The listing builds one solid part. Answer for the finished solid, in the listing's coordinates (mm). Coordinates: 2 decimals unless noted, no trailing zeros. Loops run counter-clockwise (first coordinate to the right, second up) from the corner with the lowest first, then second, coordinate; pieces in that order, holes last. Notation, with made-up numbers: (15, 3.5) - (64, 3.5) arc R33 cw to (64, 33.5) - close; hole circle Ø4 at (67.5, 52.25). An arc over 180 degrees is marked (long way). One line per question, with ' | ' between items.
from build123d import *

# Parameters (mm, degrees)
SKETCH1_R           = 13.2
SKETCH1_R_2         = 6
BOSS_EXTRUDE1_DEPTH = 6
CUT_EXTRUDE1_DEPTH  = 7


with BuildPart() as part:
    # Sketch1 → Boss-Extrude1 (new body)
    with BuildSketch(Plane.XY):
        Circle(SKETCH1_R)
        Circle(SKETCH1_R_2, mode=Mode.SUBTRACT)
    extrude(amount=BOSS_EXTRUDE1_DEPTH)

    # Sketch2 → Cut-Extrude1 (cut, through all)
    with BuildSketch(Plane.XY.offset(6)):
        with BuildLine():
            ThreePointArc((-2.819851171, 12.895287487), (0, 13.2), (2.819851171, 12.895287487))
            ThreePointArc((2.819851171, 12.895287487), (1.826256171, 11.910750525), (1.819851171, 10.512))
            ThreePointArc((1.819851171, 10.512), (0, 10.668364555), (-1.819851171, 10.512))
            ThreePointArc((-1.819851171, 10.512), (-1.826256171, 11.910750525), (-2.819851171, 12.895287487))
        make_face()
    extrude(amount=-CUT_EXTRUDE1_DEPTH, mode=Mode.SUBTRACT)


solid = part.part
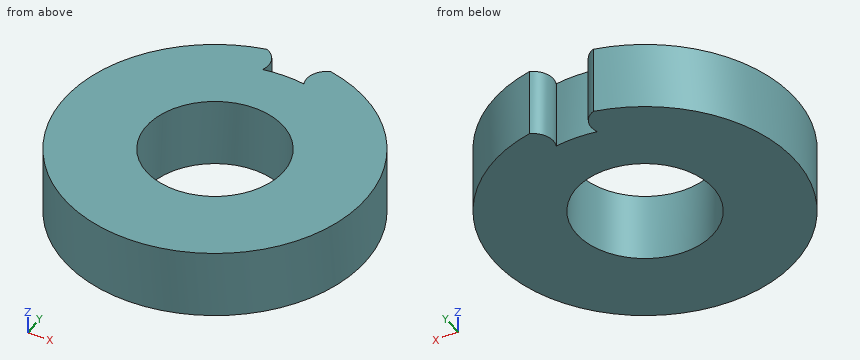
Item 1: Each of these flat-tipped pins is pushed along its axis until it touches: pin 1 Ø11 at (x, y) = (0, 0) entering from +Z; pin 2 Ø3 at (x, z) = (7, 0.5) entering from +Y; pin 3 Ø2 at (y, z) = (-4, 2) entering from -X; pin 4 Ø2 at (x, z) = (-1.5, 5) entering from +Y. Where does it stop, or does it pass through?
Taken from the geometry:
pin 1: passes through | pin 2: stops at y = 12 | pin 3: stops at x = -12.85 | pin 4: stops at y = 12.73
Item 2: Find section B-B, the plane y = 0. Write down the section's boundary in (x, z), plus the area to 3 significant figures.
Taken from the geometry:
outline: (-13.2, 0) - (-6, 0) - (-6, 6) - (-13.2, 6) - close; (6, 0) - (13.2, 0) - (13.2, 6) - (6, 6) - close | area: 86.4 mm2
Item 3: Find section D-D, the plane y = 6.75. Write down the section's boundary in (x, z), plus the area to 3 significant figures.
Taken from the geometry:
outline: (-11.34, 0) - (11.34, 0) - (11.34, 6) - (-11.34, 6) - close | area: 136 mm2
Item 4: Find section C-C, the plane z = 2.3. Write down the section's boundary in (x, y), plus the area to 3 significant figures.
Taken from the geometry:
outline: (-2.82, 12.9) arc R13.2 ccw (long way) to (2.82, 12.9) arc R1.83 ccw to (1.82, 10.51) arc R10.67 ccw to (-1.82, 10.51) arc R1.83 ccw to start; hole circle Ø12 at (0, 0) | area: 424 mm2
Item 5: Find section A-A, the plane x = 0. Write down the section's boundary in (y, z).
Taken from the geometry:
outline: (-13.2, 0) - (-6, 0) - (-6, 6) - (-13.2, 6) - close; (6, 0) - (10.67, 0) - (10.67, 6) - (6, 6) - close
Item 6: Find the intervals of material crossed by line 1 (Y direction, x = 0, z = 2.5); line 2 (X direction, y = -0.25, z = 0.3); line 3 (Y direction, x = 4.5, z = 3.3), in increasing order. Write a range as [from, to].
Taken from the geometry:
line 1: y = [-13.2, -6], [6, 10.67] | line 2: x = [-13.2, -5.99], [5.99, 13.2] | line 3: y = [-12.41, -3.97], [3.97, 12.41]
